Design review of the part built by this model. Coordinates are the model's own, in mm. A direction names the side the tool comes from. Give positions to 0.01 mm unless a question says otherwise; leave off trailing zeros. Order: outer loops, then holes, each group sorted by start corner. A loop starts at its lowest first (then second) coordinate and runs counter-clockwise, first axis right, second up. Notation, with made-up numbers: (-39, -3) -> (-5, -3) arc R21 ccw to (-5, 1) -> close; hole circle Ø2 at (-20.5, 63.25). An arc over 180 degrees is marked (long way). One line per item, written item: value. Start each with the question number.
1) Tool access review of faces 1 (the face through (-30.743, -5, 25)), 2 (the face through (33.698, -1, 22)), 3 (the face through (2, -2.1, 24)): name each direction out of +Z, -Z, +X, -X, +Y, -Y from which nothing blocks a thin tool from reaching the whole face with its end or side.
2) Wall thickness on line 1 along Y through (x, z) = (9, 24.75); line 2 along Z through (x, y) = (-4.5, -3.5); line 3 along Z through (x, y) = (29.5, -4): over which ranges is each line inside the solid? List them lowest first. Write a range as from..to.
3) Consider section D-D (z = 23.75). State the section outline as (x, y) points, plus the area to 3 significant figures.
4) Consider section C-C (y = -4). State the section outline as (x, z) points, plus the area to 3 significant figures.
5) The part is to be moulded in two halves that separate along Y. For faces 4 (the face through (-2, 0, 25)), 5 (the face through (-36.4, -9, 24)), 6 (the face through (-33.6, -3.15, 24.6)), say which applies: released by +Y, released by -Y, zero draft, split by the parting line, or undercut.
6) Consider section B-B (x = -12). State the section outline as (y, z) points.
7) Consider section A-A (y = -1). State the section outline as (x, z) points, plus the area to 3 significant figures.
8) For pin 1 (3 mm diameter, centred on x = 21, y = -6, fed in from -Z); pin 2 (2.5 mm diameter, centred on x = -32.97, z = 26.26, fed in from -Y); pin 3 (1.2 mm diameter, centred on y = -4.5, z = 24.5, fed in from -X), all flat-tipped, find the tip position at first contact; note any pin that passes through.
from build123d import *

# Parameters (mm, degrees)
F1_DEPTH = 10.3
F2_W     = 6.2
F2_H     = 4
F3_DEPTH = 29.457661
F4_R     = 1.5
F5_DEPTH = 10.301
F6_W     = 62.441146
F6_H     = 6.1
F7_DEPTH = 8


with BuildPart() as f1:
    # F0 (on Front) → F1 (new body)
    with BuildSketch(Plane.XZ):
        with BuildLine():
            Line((29.198073, 29.456661), (-33.899927, 29.456661))
            ThreePointArc((-33.899927, 29.456661), (-35.667694, 28.724428), (-36.399927, 26.956661))
            Line((-36.399927, 26.956661), (-36.399927, 19.956661))
            Line((-36.399927, 19.956661), (33.698073, 19.956661))
            Line((33.698073, 19.956661), (33.698073, 24.956661))
            ThreePointArc((33.698073, 24.956661), (32.380053, 28.138642), (29.198073, 29.456661))
        make_face()
    extrude(amount=F1_DEPTH)

    # F2 (on Top) → F3 (cut, through all)
    with BuildSketch(Plane.XY):
        with Locations((-33.843073, -5.15)):
            Rectangle(F2_W, F2_H)
    extrude(amount=F3_DEPTH, mode=Mode.SUBTRACT)

    # F4 (on Front) → F5 (cut, through all)
    with BuildSketch(Plane.XZ):
        with Locations((-32.970642, 26.256661)):
            Circle(F4_R)
    extrude(amount=F5_DEPTH, mode=Mode.SUBTRACT)

    # F6 (on face) → F7 (cut)
    with BuildSketch(Plane(origin=(0, 0, 19.956661), x_dir=(1, 0, 0), z_dir=(0, 0, -1))):
        with Locations((2.4775, 5.15)):
            Rectangle(F6_W, F6_H)
    extrude(amount=-F7_DEPTH, mode=Mode.SUBTRACT)


solid = f1.part
Checked values:
1. face 1: +Z, -Z, -X
1. face 2: +Z, -Z, +X, +Y, -Y
1. face 3: -Z, +X
2. line 1: y = -10.3..-8.2, -2.1..0
2. line 2: z = 27.96..29.46
2. line 3: z = 27.96..29.45
3. outline: (-36.4, -10.3) -> (33.7, -10.3) -> (33.7, -8.2) -> (-28.74, -8.2) -> (-28.74, -2.1) -> (33.7, -2.1) -> (33.7, 0) -> (-36.4, 0) -> (-36.4, -3.15) -> (-30.74, -3.15) -> (-30.74, -7.15) -> (-36.4, -7.15) -> close
3. area: 318 mm^2
4. outline: (-30.74, 19.96) -> (-28.74, 19.96) -> (-28.74, 27.96) -> (32.55, 27.96) arc R4.5 ccw to (29.2, 29.46) -> (-30.74, 29.46) -> close
4. area: 109 mm^2
5. face 4: released by +Y
5. face 5: zero draft
5. face 6: undercut
6. outline: (-10.3, 19.96) -> (-8.2, 19.96) -> (-8.2, 27.96) -> (-2.1, 27.96) -> (-2.1, 19.96) -> (0, 19.96) -> (0, 29.46) -> (-10.3, 29.46) -> close
7. outline: (-36.4, 19.96) -> (33.7, 19.96) -> (33.7, 24.96) arc R4.5 ccw to (29.2, 29.46) -> (-33.9, 29.46) arc R2.5 ccw to (-36.4, 26.96) -> close; hole circle Ø3 at (-32.97, 26.26)
7. area: 653 mm^2
8. pin 1: stops at z = 27.96
8. pin 2: passes through
8. pin 3: stops at x = -30.74
